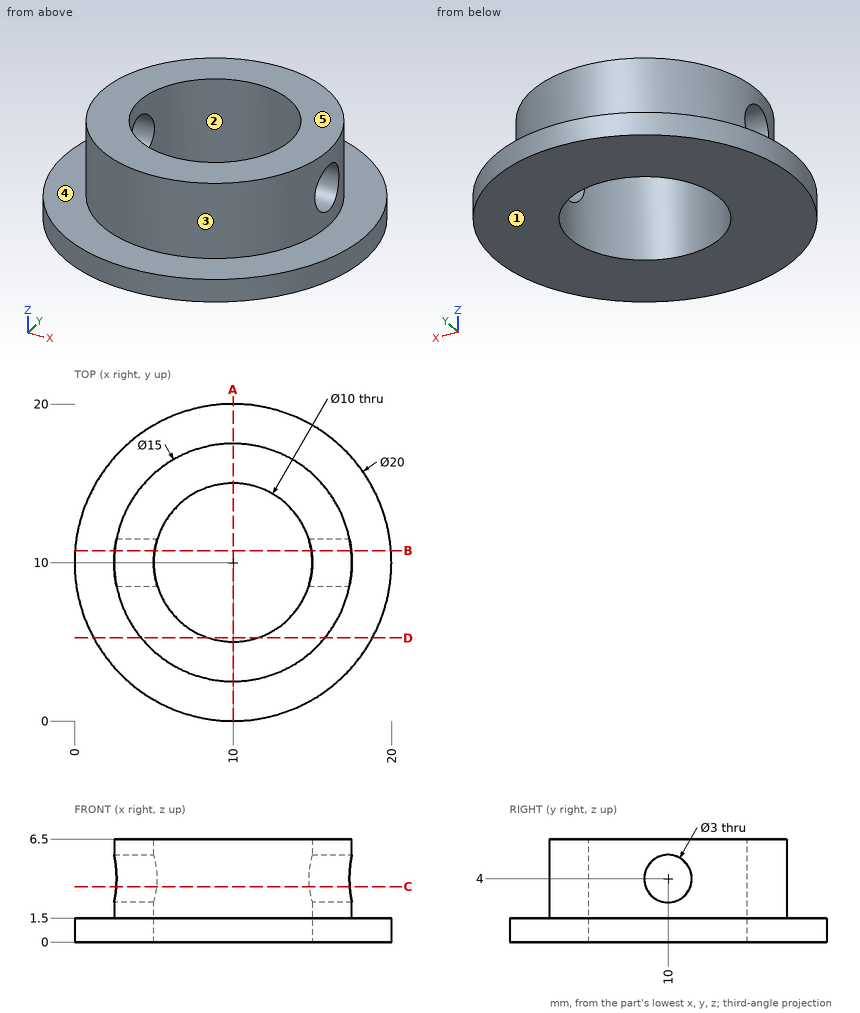
Geometry check sheet. Reference: drawing and pictorial views, mm from the part's lowest x, y, z. A direction names the side the tool comes from. Round coordinates to 2 decimals unless told otherwise and drop trailing zeros. Loops run counter-clockwise (first coordinate to the right, second up) from the corner with the lowest first, then second, coordinate; pieces in that order, holes last. Notation, with made-up numbers: (-31.75, 59.25) -> (26.25, 59.25) arc R12 ccw to (26.25, 69.25) -> close; hole circle Ø7 at (-25, 21.25). An arc over 180 degrees is marked (long way). Use a Markdown table: item, result.
(1) Sectioned sample at D-D (y = 5.25). Enter the section's corners in (x, z), then the cut area to 3 significant figures.
Calculated:
| item | result |
|---|---|
| outline | (1.2, 0) -> (8.44, 0) -> (8.44, 6.5) -> (4.2, 6.5) -> (4.2, 1.5) -> (1.2, 1.5) -> close; (11.56, 0) -> (18.8, 0) -> (18.8, 1.5) -> (15.8, 1.5) -> (15.8, 6.5) -> (11.56, 6.5) -> close |
| area | 64.1 mm² |
(2) Scan lines: probe 1 along Y at (x, z) = (10, 4); probe 2 along Z at (x, y) = (16.75, 10). Record each from-to range of solid material in increasing order.
Calculated:
| item | result |
|---|---|
| probe 1 | 2.5 to 5, 15 to 17.5 |
| probe 2 | 0 to 2.5, 5.5 to 6.5 |
(3) Sectioned sample at B-B (y = 10.75). Enter the section's corners in (x, z), then the cut area to 3 significant figures.
Calculated:
| item | result |
|---|---|
| outline | (0.03, 0) -> (5.06, 0) -> (5.06, 2.7) -> (2.54, 2.7) -> (2.54, 1.5) -> (0.03, 1.5) -> close; (2.54, 5.3) -> (5.06, 5.3) -> (5.06, 6.5) -> (2.54, 6.5) -> close; (14.94, 0) -> (19.97, 0) -> (19.97, 1.5) -> (17.46, 1.5) -> (17.46, 2.7) -> (14.94, 2.7) -> close; (14.94, 5.3) -> (17.46, 5.3) -> (17.46, 6.5) -> (14.94, 6.5) -> close |
| area | 27.2 mm² |
(4) Go/stop test with flat-tipped pins: P1, Ø3, axis at x = 14, y = 8, coming from the -Z side; P2, Ø1.5, axis at x = 2.5, z = 5, coming from the -Y side; P3, Ø2, axis at x = 15.5, z = 3, coming from the +Y side; P4, Ø3.5, axis at y = 10, z = 4, coming from the -X side. Record where each tip stops, or that it passes through.
Calculated:
| item | result |
|---|---|
| P1 | z = 0 |
| P2 | y = 6.73 |
| P3 | y = 16 |
| P4 | x = 2.5 |
(5) Sectioned sample at A-A (x = 10). Enter the section's corners in (y, z).
Calculated:
| item | result |
|---|---|
| outline | (0, 0) -> (5, 0) -> (5, 6.5) -> (2.5, 6.5) -> (2.5, 1.5) -> (0, 1.5) -> close; (15, 0) -> (20, 0) -> (20, 1.5) -> (17.5, 1.5) -> (17.5, 6.5) -> (15, 6.5) -> close |
(6) Set-up check for the marked faces 4 and 5: record each of +Z, -Z, +X, -X, +Y, -Y from which the full face is reachable in a straight line by a thin tool's end or side.
Calculated:
| item | result |
|---|---|
| face 4 | +Z |
| face 5 | +Z, +X, -X, +Y, -Y |
(7) Mould release check, pull along Y, two halves, no side actions. Record for the marked faces 1, 2 and 3: released by +Y, released by -Y, zero draft, split by the parting line, or undercut.
Calculated:
| item | result |
|---|---|
| face 1 | zero draft |
| face 2 | undercut |
| face 3 | split by the parting line |
(8) Sectioned sample at C-C (z = 3.5). Enter the section's corners in (x, y), then the cut area to 3 significant figures.
Calculated:
| item | result |
|---|---|
| outline | (2.63, 8.59) arc R7.5 ccw to (17.37, 8.59) -> (14.8, 8.59) arc R5 cw to (5.2, 8.59) -> close; (2.63, 11.41) -> (5.2, 11.41) arc R5 cw to (14.8, 11.41) -> (17.37, 11.41) arc R7.5 ccw to start |
| area | 83.9 mm² |
